The figure shows three views and two pictorial views of one solid part (mm, origin at its lowest corner). Answer the questions. A direction names the side the tool comes from. Coordinates: 2 decimals unless noted, no trailing zeros. Order: outer loops, then holes, each group sorted by start corner. A loop starts at its lowest first (then second) coordinate and runs counter-clockwise, first axis right, second up. Notation, with made-up numbers: (70, -31) -> (113, -31) arc R16 cw to (113, -13) -> close; hole circle Ø8 at (-19, -40). An arc over 180 degrees is marked (long way). Return JSON: item names as keys, results as strings.
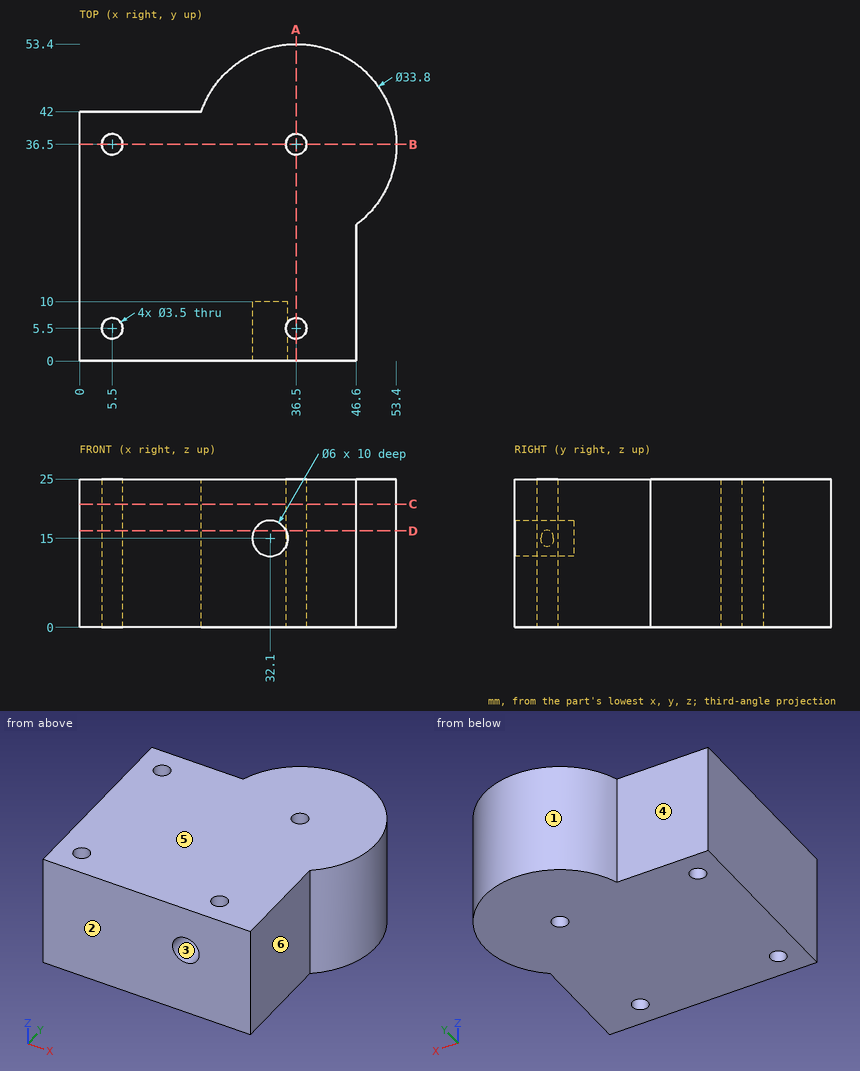
Item 1: The part is cut by section D-D on z = 16.25. Determine the outline of the cut face in (x, y), plus the area to 3 significant figures.
Answer list:
{"outline": "(0, 0) -> (29.37, 0) -> (29.37, 10) -> (34.83, 10) -> (34.83, 6.01) arc R1.75 cw (long way) to (34.83, 4.99) -> (34.83, 0) -> (46.6, 0) -> (46.6, 22.95) arc R16.9 ccw (long way) to (20.52, 42) -> (0, 42) -> close; hole circle Ø3.5 at (5.5, 5.5); hole circle Ø3.5 at (5.5, 36.5); hole circle Ø3.5 at (36.5, 36.5)", "area": "2,230 mm2"}
Item 2: The part is cut by section A-A on x = 36.5. Determine the outline of the cut face in (y, z), plus the area to 3 significant figures.
Answer list:
{"outline": "(0, 0) -> (3.75, 0) -> (3.75, 25) -> (0, 25) -> close; (7.25, 0) -> (34.75, 0) -> (34.75, 25) -> (7.25, 25) -> close; (38.25, 0) -> (53.4, 0) -> (53.4, 25) -> (38.25, 25) -> close", "area": "1,160 mm2"}
Item 3: Find the intervals of material crossed by probe 1 along Y at (x, z) = (5.5, 14.25); probe 2 along Y at (x, z) = (36.5, 18.5); probe 3 along Z at (x, y) = (32, 2), in increasing order.
Answer list:
{"probe 1": "0 to 3.75, 7.25 to 34.75, 38.25 to 42", "probe 2": "0 to 3.75, 7.25 to 34.75, 38.25 to 53.4", "probe 3": "0 to 12, 18 to 25"}
Item 4: Which of the six approach directions +Z, -Z, +X, -X, +Y, -Y give full straight-line access (tool end or side, diameter ignored) to the marked faces 4, 5 and 6?
Answer list:
{"face 4": "+Z, -Z, -X, +Y", "face 5": "+Z, +X, -X, +Y, -Y", "face 6": "+Z, -Z, +X, -Y"}
Item 5: Flat-ended cylindrical pins translate along their axes: pin 1 (1 mm diameter, centred on x = 24, z = 21, fed in from +Y); pin 2 (12 mm diameter, centred on y = 17.5, z = 17, fed in from +X); pin 3 (8 mm diameter, centred on y = 21, z = 4, fed in from +X); pin 4 (3 mm diameter, centred on x = 36.5, y = 36.5, fed in from +Z). Find the tip coordinate at first contact, or state that the pin passes through.
Answer list:
{"pin 1": "y = 48.4", "pin 2": "x = 47.3", "pin 3": "x = 48.88", "pin 4": "through"}
Item 6: Determine the mould class of the marked faces 1, 2 and 3 for opening direction X: pulls with the +X half, pulls with the -X half, needs draft (parallel to the pull), parting line crosses it, or undercut.
Answer list:
{"face 1": "parting line crosses it", "face 2": "needs draft", "face 3": "undercut"}
Item 7: The part is cut by section C-C on z = 20.75. Determine the outline of the cut face in (x, y).
Answer list:
{"outline": "(0, 0) -> (46.6, 0) -> (46.6, 22.95) arc R16.9 ccw (long way) to (20.52, 42) -> (0, 42) -> close; hole circle Ø3.5 at (5.5, 5.5); hole circle Ø3.5 at (5.5, 36.5); hole circle Ø3.5 at (36.5, 5.5); hole circle Ø3.5 at (36.5, 36.5)"}
